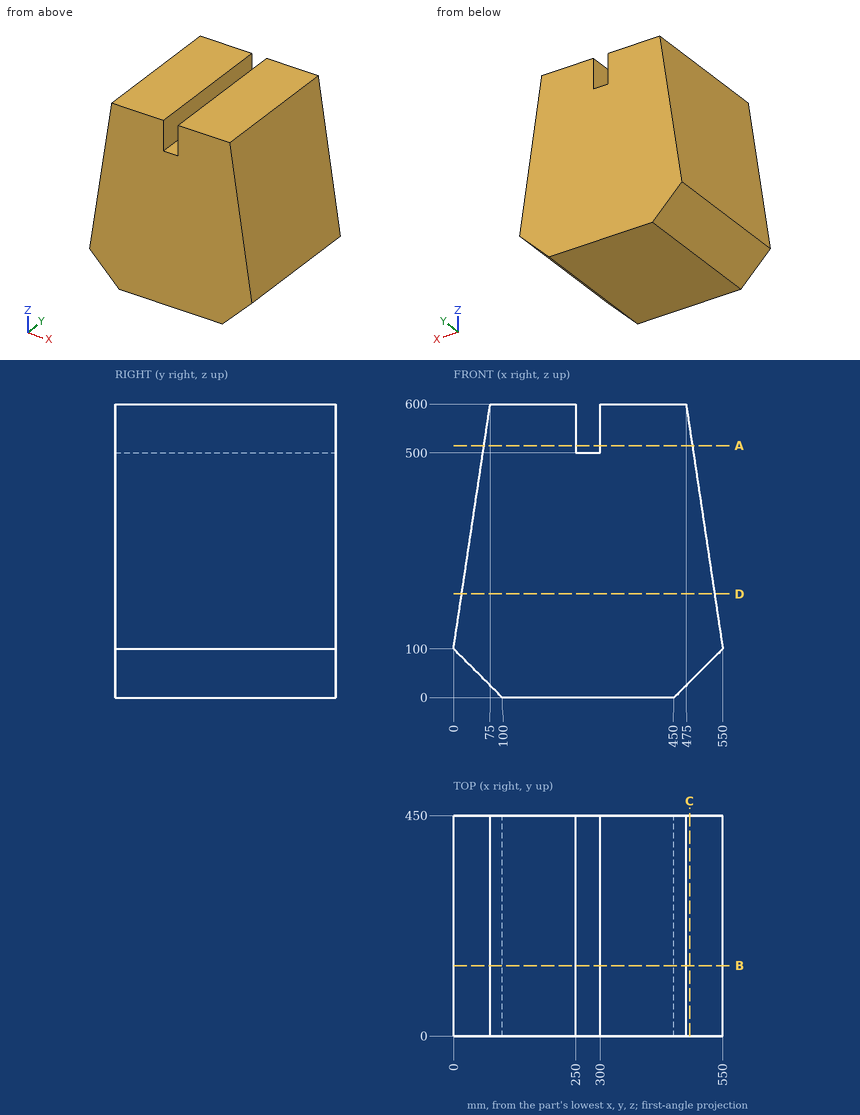
Can you work these out from the drawing? Everything is in mm from the part's minimum corner. Round coordinates to 2 decimals unless told otherwise and drop trailing zeros. Loops run counter-clockwise (first coordinate to the right, second up) from the corner with the lowest first, then second, coordinate; pieces in that order, holes last. Notation, with made-up numbers: (50.25, 14) -> (67.25, 14) arc R13 ccw to (67.25, 26) -> close; hole circle Ø5 at (43, -23.5). An arc over 180 degrees is marked (long way). Answer in a Markdown table with one row per item.
Item 1: Suppose I cut it at A-A, the plane z = 515. List the corners of the cut face in (x, y) for me, plus the area to 3 significant figures.
Answer block:
| item | result |
|---|---|
| outline | (62.25, 0) -> (250, 0) -> (250, 450) -> (62.25, 450) -> close; (300, 0) -> (487.75, 0) -> (487.75, 450) -> (300, 450) -> close |
| area | 169,000 mm² |
Item 2: Will these pins go through, and if not, where does the flat tip stop? P1, Ø2, axis at x = 393.5, y = 112, coming from the -Z side; P2, Ø10, axis at y = 387, z = 371, coming from the +X side; P3, Ø6, axis at y = 253.5, z = 416, coming from the -X side.
Answer block:
| item | result |
|---|---|
| P1 | z = 0 |
| P2 | x = 510.1 |
| P3 | x = 46.95 |
Item 3: Suppose I cut it at C-C, the plane x = 482.5. List the corners of the cut face in (y, z) for me.
Answer block:
| item | result |
|---|---|
| outline | (0, 32.5) -> (450, 32.5) -> (450, 550) -> (0, 550) -> close |
Item 4: If I drill on probe 1 along X at (y, z) = (60, 54); probe 2 along X at (y, z) = (334.5, 184.5) (3 decimals), over which ranges is the centre line in solid material (lowest first)?
Answer block:
| item | result |
|---|---|
| probe 1 | 46 to 504 |
| probe 2 | 12.675 to 537.325 |
Item 5: Suppose I cut it at B-B, the plane y = 143.5. List the corners of the cut face in (x, z) for me.
Answer block:
| item | result |
|---|---|
| outline | (0, 100) -> (100, 0) -> (450, 0) -> (550, 100) -> (475, 600) -> (300, 600) -> (300, 500) -> (250, 500) -> (250, 600) -> (75, 600) -> close |
Item 6: Suppose I cut it at D-D, the plane z = 212. List the corners of the cut face in (x, y) for me, plus the area to 3 significant figures.
Answer block:
| item | result |
|---|---|
| outline | (16.8, 0) -> (533.2, 0) -> (533.2, 450) -> (16.8, 450) -> close |
| area | 232,000 mm² |
